from build123d import *

# Parameters (mm, degrees)
ESQUISSE1_R                  = 8.1
ESQUISSE1_R_2                = 1.65
BOSS_EXTRU_1_DEPTH           = 4
ESQUISSE2_W                  = 50
ESQUISSE2_H                  = 5
BOSS_EXTRU_2_DEPTH           = 80
BOSS_EXTRU_3_DEPTH           = 20
ENL_V_MAT_EXTRU_2_DEPTH      = 99.748417709
ENL_V_MAT_EXTRU_2_DEPTH_BACK = 99.748417709
CHANFREIN1_SIZE              = 3
CHANFREIN2_SIZE              = 2
BOSS_EXTRU_4_DEPTH           = 4
BOSS_EXTRU_4_DEPTH_BACK      = 4
CHANFREIN3_SIZE              = 5
ENL_V_MAT_EXTRU_3_DEPTH      = 5
ENL_V_MAT_EXTRU_3_DEPTH_BACK = 20
ESQUISSE6_R                  = 1.25
CONG_1_R                     = 3


with BuildPart() as part:
    # Esquisse1 → Boss.-Extru.1 (new body)
    with BuildSketch(Plane.XY):
        with BuildLine():
            Line((-25, -20), (-25, -25))
            Line((-25, -25), (25, -25))
            Line((25, -25), (25, -20))
            Line((25, -20), (19.512195122, 4.390243902))
            ThreePointArc((19.512195122, 4.390243902), (0, 20), (-19.512195122, 4.390243902))
            Line((-19.512195122, 4.390243902), (-25, -20))
        make_face()
        Circle(ESQUISSE1_R, mode=Mode.SUBTRACT)
        with Locations((-10.25, 5.917840259)):
            Circle(ESQUISSE1_R_2, mode=Mode.SUBTRACT)
        with Locations((10.25, 5.917840259)):
            Circle(ESQUISSE1_R_2, mode=Mode.SUBTRACT)
        with Locations((0, -11.835680518)):
            Circle(ESQUISSE1_R_2, mode=Mode.SUBTRACT)
    extrude(amount=BOSS_EXTRU_1_DEPTH)

    # Esquisse2 → Boss.-Extru.2 (add)
    with BuildSketch(Plane.XY.offset(4)):
        with Locations((0, -22.5)):
            Rectangle(ESQUISSE2_W, ESQUISSE2_H)
    extrude(amount=BOSS_EXTRU_2_DEPTH)

    # Esquisse4 → Boss.-Extru.3 (add)
    with BuildSketch(Plane.XY.offset(4)):
        Polygon((-20.5, 0), (-20.5, -20), (-25, -20), align=None)
        Polygon((20.5, -20), (25, -20), (20.5, 0), align=None)
    extrude(amount=BOSS_EXTRU_3_DEPTH)

    # Esquisse5 → Enlèv. mat.-Extru.2 (cut, two sides: drawn at the far end of the back side and taken through both)
    with BuildSketch(Plane(origin=(-20.5, 0, 0), x_dir=(0, 0, -1), z_dir=(1, 0, 0)).offset(-ENL_V_MAT_EXTRU_2_DEPTH_BACK)):
        Polygon((-4, 0), (-24, 0), (-24, -20), (-10, -6), (-4, -6), align=None)
    extrude(amount=ENL_V_MAT_EXTRU_2_DEPTH + ENL_V_MAT_EXTRU_2_DEPTH_BACK, mode=Mode.SUBTRACT)

    # Chanfrein1
    chanfrein1_edges = [part.edges().sort_by_distance(p)[0] for p in [
        (-20.5, -13, 4),
        (-20.5, -20, 14),
        (0, -20, 4),
        (20.5, -20, 14),
        (20.5, -13, 4),
    ]]
    chamfer(chanfrein1_edges, length=CHANFREIN1_SIZE)

    # Chanfrein2
    chanfrein2_edges = [part.edges().sort_by_distance(p)[0] for p in [
        (-19.675, -6, 4),
        (19.675, -6, 4),
    ]]
    chamfer(chanfrein2_edges, length=CHANFREIN2_SIZE)

    # Esquisse7 → Boss.-Extru.4 (add, two sides: drawn at the far end of the back side and taken through both)
    with BuildSketch(Plane.XY.offset(46).offset(-BOSS_EXTRU_4_DEPTH_BACK)):
        with BuildLine():
            Line((-15, 0), (-20.456097561, 0.195121951))
            Line((-20.456097561, 0.195121951), (-25, -20))
            Line((-25, -20), (25, -20))
            Line((25, -20), (20.5, 0))
            Line((20.5, 0), (15, 0))
            ThreePointArc((15, 0), (0, -15), (-15, 0))
        make_face()
    extrude(amount=BOSS_EXTRU_4_DEPTH + BOSS_EXTRU_4_DEPTH_BACK)

    # Chanfrein3
    # the kernel refuses this chamfer: 5 mm, written as the material it adds along each edge
    with BuildSketch(Plane(origin=(-25, -20, 42), x_dir=(0, -0.027495876610586317, -0.9996219169112968), z_dir=(1, 0, 0))) as chanfrein3_piece_1_section:
        Polygon((CHANFREIN3_SIZE * 0.999621916911, CHANFREIN3_SIZE * 0.0274958766106), (-CHANFREIN3_SIZE * 0.0274958766106, CHANFREIN3_SIZE * 0.999621916911), (0, 0), align=None)
    chanfrein3_piece_1 = extrude(amount=50, mode=Mode.PRIVATE)
    chanfrein3_piece_1 = split(chanfrein3_piece_1, bisect_by=Plane(origin=(23.445378938, -13.090573058, 40.343175913), z_dir=(-0.9756097560975611, -0.2195121951219509, 0)), keep=Keep.TOP, mode=Mode.PRIVATE)
    chanfrein3_piece_1 = split(chanfrein3_piece_1, bisect_by=Plane(origin=(-23.445378938, -13.090573058, 40.343175913), z_dir=(0.9756097560975611, -0.21951219512195103, 0)), keep=Keep.TOP, mode=Mode.PRIVATE)
    chanfrein3_piece_1 = chanfrein3_piece_1 - Plane(origin=(0, 0, 40.343175913), x_dir=(1, 0, 0), z_dir=(0, 0, -1)) * Cylinder(15, 120, mode=Mode.PRIVATE)
    add(chanfrein3_piece_1)
    with BuildSketch(Plane(origin=(-25, -20, 50), x_dir=(0, -0.027495876610586317, 0.9996219169112968), z_dir=(1, 0, 0))) as chanfrein3_piece_2_section:
        Polygon((CHANFREIN3_SIZE * 0.999621916911, -CHANFREIN3_SIZE * 0.0274958766106), (-CHANFREIN3_SIZE * 0.0274958766106, -CHANFREIN3_SIZE * 0.999621916911), (0, 0), align=None)
    chanfrein3_piece_2 = extrude(amount=50, mode=Mode.PRIVATE)
    chanfrein3_piece_2 = split(chanfrein3_piece_2, bisect_by=Plane(origin=(23.445378938, -13.090573058, 51.656824087), z_dir=(-0.9756097560975611, -0.2195121951219509, 0)), keep=Keep.TOP, mode=Mode.PRIVATE)
    chanfrein3_piece_2 = split(chanfrein3_piece_2, bisect_by=Plane(origin=(-23.445378938, -13.090573058, 51.656824087), z_dir=(0.9756097560975611, -0.21951219512195103, 0)), keep=Keep.TOP, mode=Mode.PRIVATE)
    chanfrein3_piece_2 = chanfrein3_piece_2 - Plane(origin=(0, 0, 51.656824087), x_dir=(1, 0, 0), z_dir=(0, 0, -1)) * Cylinder(15, 120, mode=Mode.PRIVATE)
    add(chanfrein3_piece_2)

    # Esquisse6 → Enlèv. mat.-Extru.3 (cut, two sides: drawn at the far end of the back side and taken through both)
    with BuildSketch(Plane(origin=(0, -20, 0), x_dir=(1, 0, 0), z_dir=(0, 1, 0)).offset(-ENL_V_MAT_EXTRU_3_DEPTH_BACK)):
        with Locations(Location((-15, -74, 0), (0, 0, 90))):
            Circle(ESQUISSE6_R)
        with Locations(Location((15, -74, 0), (0, 0, 90))):
            Circle(ESQUISSE6_R)
        with Locations(Location((15, -14, 0), (0, 0, 90))):
            Circle(ESQUISSE6_R)
        with Locations(Location((-15, -14, 0), (0, 0, 90))):
            Circle(ESQUISSE6_R)
        with Locations(Location((-15, -44, 0), (0, 0, 270))):
            Circle(ESQUISSE6_R)
        with Locations(Location((15, -44, 0), (0, 0, 90))):
            Circle(ESQUISSE6_R)
    extrude(amount=ENL_V_MAT_EXTRU_3_DEPTH + ENL_V_MAT_EXTRU_3_DEPTH_BACK, mode=Mode.SUBTRACT)

    # Congé1
    cong_1_edges = [part.edges().sort_by_distance(p)[0] for p in [
        (-15, 0, 46),
        (15, 0, 46),
    ]]
    fillet(cong_1_edges, radius=CONG_1_R)


solid = part.part
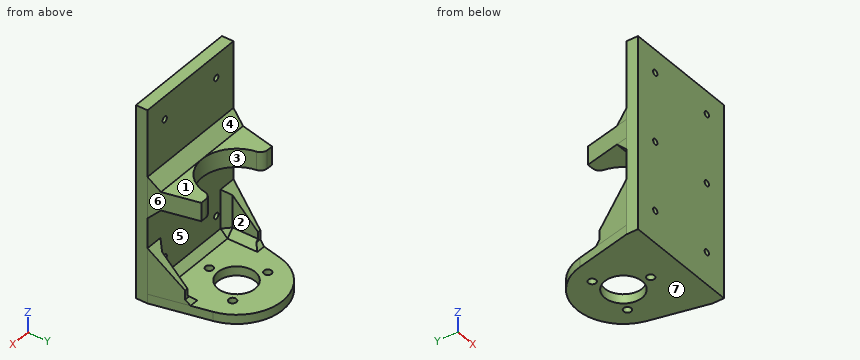
Design review of the part built by this model. Coordinates are the model's own, in mm. Face numbers are marked on the shaded views. A direction names the side the tool comes from. Coordinates: 2 decimals unless noted, no trailing zeros. Order: outer loops, then holes, each group sorted by start corner. A loop starts at its lowest first (then second) coordinate and runs counter-clockwise, first axis right, second up. Notation, with made-up numbers: (-6.75, 87) - (40.25, 87) arc R11 ccw to (40.25, 99) - close; hole circle Ø5 at (26.5, 51.5). An arc over 180 degrees is marked (long way). Put each result on its own line as item: value.
1) Take a section at D-D, the plane z = 44. Give the boundary of the cut face in (x, y), and give its area (3 significant figures).
Response values:
outline: (-25, -25) - (-16.25, -25) - (-16.25, -15) - (-13.75, -15) - (-13.75, -25) - (13.75, -25) - (13.75, -15) - (16.25, -15) - (16.25, -25) - (25, -25) - (25, -20) - (20.5, 0) - (17.75, 0) arc R3 ccw to (14.79, -2.5) arc R15 cw to (-14.8, -2.42) arc R3 ccw to (-17.66, 0.1) - (-20.46, 0.2) - (-25, -20) - close
area: 754 mm²
2) Take a section at A-A, the plane z = 14. Give the boundary of the cut face in (x, y).
Response values:
outline: (-25, -25) - (-16.25, -25) - (-16.25, -20) - (-17.5, -20) - (-20.5, -17) - (-20.5, -10) - (-22.75, -10) - (-25, -20) - close; (-13.75, -25) - (13.75, -25) - (13.75, -20) - (-13.75, -20) - close; (16.25, -25) - (25, -25) - (25, -20) - (22.75, -10) - (20.5, -10) - (20.5, -17) - (17.5, -20) - (16.25, -20) - close
3) The part is to be moulded in two halves that separate along Z. For the marked faces 4, 5, 6 and 7, say which applies: released by +Z, released by -Z, zero draft, split by the parting line, or undercut.
Response values:
face 4: released by +Z
face 5: undercut
face 6: zero draft
face 7: released by -Z
4) Wall thickness on L1, parallel to X at y = -21, z = 44; L2, parallel to Z at x = -12.5, y = -14; L3, parallel to Y at x = -21.5, z = 57.5: over which ranges is each line inside the solid? List them lowest first. Write a range as from..to.
Response values:
L1: x = -25..-16.25, -13.75..13.75, 16.25..25
L2: z = 0..4, 42..50
L3: y = -25..-20
5) Tool access review of the marked faces 1, 2 and 3: name each direction out of +Z, -Z, +X, -X, +Y, -Y from which nothing blocks a thin tool from reaching the whole face with its end or side.
Response values:
face 1: +Z, +X, -X, +Y
face 2: +Y
face 3: +Z, +Y
6) Take a section at B-B, the plane x = -10.25. Give the boundary of the cut face in (y, z).
Response values:
outline: (-25, 0) - (4.27, 0) - (4.27, 4) - (-17, 4) - (-20, 7) - (-20, 37) - (-15, 42) - (-10.95, 42) - (-10.95, 50) - (-15, 50) - (-20, 55) - (-20, 84) - (-25, 84) - close; (7.57, 0) - (17.17, 0) - (17.17, 4) - (7.57, 4) - close
7) Insertion check: P1, Ø4, axis at y = -9.5, z = 41.5, coming from the -X side; P2, Ø1.5, axis at x = -15, z = 14, coming from the +Y side; P3, Ø24, axis at x = -7.5, z = 17, coming from the +Y side; P4, Ø12, axis at x = 10, y = -10, coming from the +Z side. Each pin has a flat end and moves straight along its axis. Give the tip position at first contact, or say it passes through.
Response values:
P1: stops at x = -23.07
P2: passes through
P3: stops at y = -18
P4: stops at z = 51
8) Take a section at C-C, the plane y = -1.5. Give the boundary of the cut face in (x, z).
Response values:
outline: (-20.84, 0) - (-7.96, 0) - (-7.96, 4) - (-20.84, 4) - close; (-20.84, 42) - (-15.11, 42) - (-15.11, 50) - (-20.84, 50) - close; (7.96, 0) - (20.84, 0) - (20.84, 4) - (7.96, 4) - close; (15.15, 42) - (20.84, 42) - (20.84, 50) - (15.15, 50) - close
